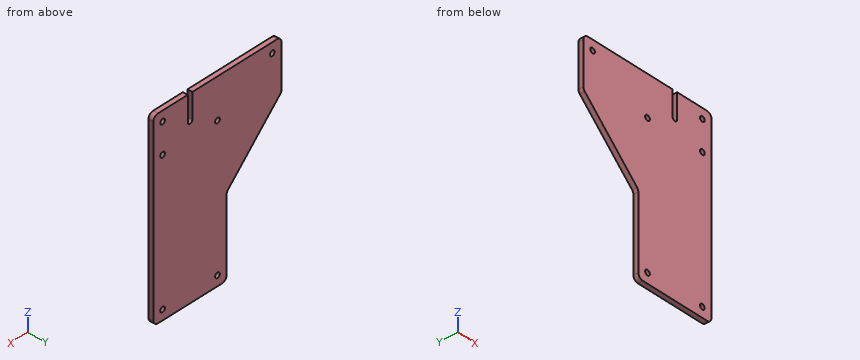
```python
from build123d import *

# Parameters (mm, degrees)
BOSS_EXTRUDE1_DEPTH         = 6.35
F_1_4_CLEARANCE_HOLE1_D     = 6.5278
F_1_4_CLEARANCE_HOLE1_DEPTH = 6.35
F_1_4_CLEARANCE_HOLE1_TIP   = 1.961148974
FILLET1_R                   = 6.35
CUT_EXTRUDE1_REACH          = 8.35


with BuildPart() as part:
    # Sketch1 → Boss-Extrude1 (new body)
    with BuildSketch(Plane(origin=(0, 0, 0), x_dir=(1, 0, 0), z_dir=(0, 1, 0))):
        Polygon((-12.7, 228.6), (88.9, 228.6), (88.9, -12.7), (-88.9, -12.7), (-88.9, 50.8), (-12.7, 127), align=None)
    extrude(amount=BOSS_EXTRUDE1_DEPTH)

    # 1/4 Clearance Hole1
    with Locations(Plane(origin=(0, 6.35, 0), x_dir=(1, 0, 0), z_dir=(0, 1, 0))):
        with Locations((76.2, 215.9), (0, 215.9), (0, 38.1), (76.2, 38.1), (76.2, 0), (-76.2, 0)):
            Hole(F_1_4_CLEARANCE_HOLE1_D / 2, depth=F_1_4_CLEARANCE_HOLE1_DEPTH)
            with Locations((0, 0, -(F_1_4_CLEARANCE_HOLE1_DEPTH + F_1_4_CLEARANCE_HOLE1_TIP / 2))):  # 118° drill point
                Cone(0, F_1_4_CLEARANCE_HOLE1_D / 2, F_1_4_CLEARANCE_HOLE1_TIP, mode=Mode.SUBTRACT)

    # Fillet1
    fillet1_edges = [part.edges().sort_by_distance(p)[0] for p in [
        (-12.7, 3.175, -228.6),
        (88.9, 3.175, -228.6),
        (88.9, 3.175, 12.7),
        (-88.9, 3.175, 12.7),
        (-88.9, 3.175, -50.8),
        (-12.7, 3.175, -127),
    ]]
    fillet(fillet1_edges, radius=FILLET1_R)

    # Sketch4 → Cut-Extrude1 (cut, up to next)
    with BuildSketch(Plane(origin=(0, 6.35, 0), x_dir=(1, 0, 0), z_dir=(0, 1, 0)), mode=Mode.PRIVATE) as cut_extrude1_sk1:
        with BuildLine():
            Line((41.275, 19.05), (41.275, -12.7))
            ThreePointArc((41.275, -12.7), (38.1, -15.875), (34.925, -12.7))
            Line((34.925, -12.7), (34.925, 19.05))
            ThreePointArc((34.925, 19.05), (38.1, 22.225), (41.275, 19.05))
        make_face()
    cut_extrude1_tool1 = extrude(cut_extrude1_sk1.sketch, amount=-CUT_EXTRUDE1_REACH, mode=Mode.PRIVATE) & part.part
    add(cut_extrude1_tool1.solids().sort_by_distance((38.1, 6.35, -3.175))[0], mode=Mode.SUBTRACT)


solid = part.part
```
Verification items for the finished model (mm, model axes). Round coordinates to 2 decimals unless told otherwise and drop trailing zeros. Order: outer loops, then holes, each group sorted by start corner. A loop starts at its lowest first (then second) coordinate and runs counter-clockwise, first axis right, second up.
1) Cross-section at C-C, the plane z = 0. Record the cut outline in (x, y) (3 decimals), plus the area to 3 significant figures.
Geometry says:
outline: (-88.9, 0) - (-79.464, 0) - (-79.464, 6.35) - (-88.9, 6.35) - close; (-72.936, 0) - (34.925, 0) - (34.925, 6.35) - (-72.936, 6.35) - close; (41.275, 0) - (72.936, 0) - (72.936, 6.35) - (41.275, 6.35) - close; (79.464, 0) - (88.9, 0) - (88.9, 6.35) - (79.464, 6.35) - close
area: 1,010 mm2
2) Depth check by flat-ended pin: pin 1 (10.5 mm diameter, centred on x = 0, z = -215.9, fed in from +Y); pin 2 (1 mm diameter, centred on y = 1.5, z = -192.5, fed in from -X). Enter the tip coordinate at first touch or a pass-through.
Geometry says:
pin 1: stops at y = 6.35
pin 2: stops at x = -12.7
3) Cross-section at B-B, the plane x = 76.2. Record the cut outline in (y, z), plus the area to 3 significant figures.
Geometry says:
outline: (0, -228.6) - (6.35, -228.6) - (6.35, -219.16) - (0, -219.16) - close; (0, -212.64) - (6.35, -212.64) - (6.35, -41.36) - (0, -41.36) - close; (0, -34.84) - (6.35, -34.84) - (6.35, -3.26) - (0, -3.26) - close; (0, 3.26) - (6.35, 3.26) - (6.35, 12.7) - (0, 12.7) - close
area: 1,410 mm2
4) Cross-section at D-D, the plane x = -76.2. Record the cut outline in (y, z).
Geometry says:
outline: (0, -63.5) - (6.35, -63.5) - (6.35, -3.26) - (0, -3.26) - close; (0, 3.26) - (6.35, 3.26) - (6.35, 12.7) - (0, 12.7) - close
5) Cross-section at A-A, the plane z = -38.1. Record the cut outline in (x, y).
Geometry says:
outline: (-88.9, 0) - (-3.26, 0) - (-3.26, 6.35) - (-88.9, 6.35) - close; (3.26, 0) - (72.94, 0) - (72.94, 6.35) - (3.26, 6.35) - close; (79.46, 0) - (88.9, 0) - (88.9, 6.35) - (79.46, 6.35) - close
6) Material ranges on line 1 (Z direction, x = 0, y = 2.25); line 2 (Z direction, x = 76.2, y = 2.25); line 3 (X direction, y = 1.5, z = -38.1), recorded low to high.
Geometry says:
line 1: z = -228.6 to -219.16, -212.64 to -41.36, -34.84 to 12.7
line 2: z = -228.6 to -219.16, -212.64 to -41.36, -34.84 to -3.26, 3.26 to 12.7
line 3: x = -88.9 to -3.26, 3.26 to 72.94, 79.46 to 88.9
